Geometry check sheet. Reference: drawing and pictorial views, mm from the part's lowest x, y, z. A direction names the side the tool comes from. Round coordinates to 2 decimals unless told otherwise and drop trailing zeros. Loops run counter-clockwise (first coordinate to the right, second up) from the corner with the lowest first, then second, coordinate; pieces in that order, holes last. Notation, with made-up numbers: (45, -1.5) -> (92, -1.5) arc R14 ccw to (92, 16.5) -> close; hole circle Ø9 at (-35, 7). An arc over 180 degrees is marked (long way). Write item = value, one per line.
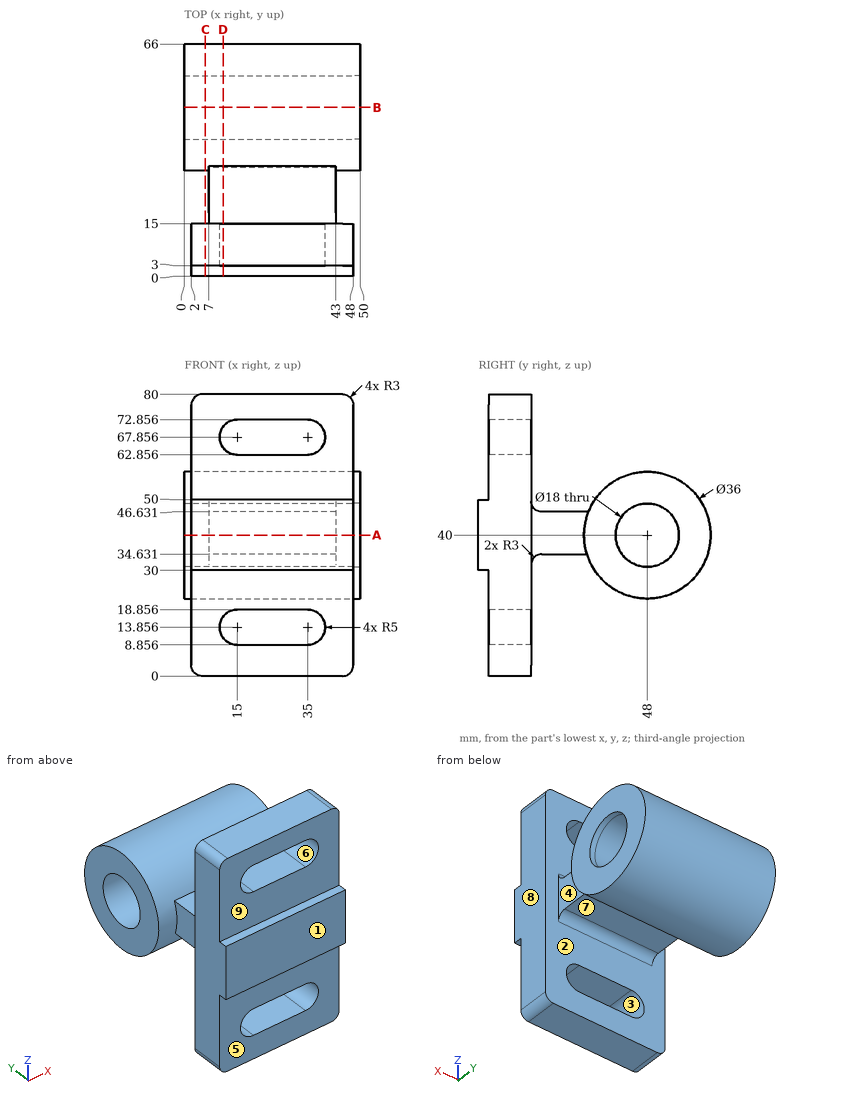
(1) Draft check along Y on the marked faces 1, 2, 3 and 4. Enter one of: released by +Y, released by -Y, zero draft, split by the parting line, or undercut.
Filled sheet:
face_1 = released by -Y
face_2 = undercut
face_3 = zero draft
face_4 = undercut
(2) Sectioned sample at A-A, the plane z = 40. Record the cut outline in (x, y), and give its area (3 significant figures).
Filled sheet:
outline = (0, 30) -> (7, 30) -> (7, 15) -> (2, 15) -> (2, 0) -> (48, 0) -> (48, 15) -> (43, 15) -> (43, 30) -> (50, 30) -> (50, 39) -> (0, 39) -> close; (0, 57) -> (50, 57) -> (50, 66) -> (0, 66) -> close
area = 2,130 mm2
(3) Set-up check for the marked faces 5, 6, 7, 8 and 9: record each of +Z, -Z, +X, -X, +Y, -Y from which the full face is reachable in a straight line by a thin tool's end or side.
Filled sheet:
face_5 = -Z, +X, -X, -Y
face_6 = +Y, -Y
face_7 = -Z, +X, -X
face_8 = +Z, -Z, +X, -Y
face_9 = +Z, +X, -X, -Y
(4) Sectioned sample at B-B, the plane y = 48. Record the cut outline in (x, z).
Filled sheet:
outline = (0, 22) -> (50, 22) -> (50, 31) -> (0, 31) -> close; (0, 49) -> (50, 49) -> (50, 58) -> (0, 58) -> close
(5) Material ranges on probe 1 along Y at (x, z) = (17, 40); probe 2 along Z at (x, y) = (17, 48); probe 3 along Y at (x, z) = (49.1, 40), recorded low to high. Write a range as from..to.
Filled sheet:
probe_1 = 0..39, 57..66
probe_2 = 22..31, 49..58
probe_3 = 30..39, 57..66
(6) Go/stop test with flat-tipped pins: pin 1 Ø13 at (y, z) = (22, 38.5) entering from -X; pin 2 Ø24 at (x, z) = (33.5, 21) entering from -Y; pin 3 Ø12 at (y, z) = (8.5, 41.5) entering from -X; pin 4 Ø23 at (x, z) = (34, 54) entering from +Y (1 decimal). Record where each tip stops, or that it passes through.
Filled sheet:
pin_1 = 7
pin_2 = 0
pin_3 = 2
pin_4 = 65.8
(7) Sectioned sample at C-C, the plane x = 6. Record the cut outline in (y, z), and give its area (3 significant figures).
Filled sheet:
outline = (0, 30) -> (3, 30) -> (3, 0) -> (15, 0) -> (15, 80) -> (3, 80) -> (3, 50) -> (0, 50) -> close; circle Ø36 at (48, 40); hole circle Ø18 at (48, 40)
area = 1,780 mm2
(8) Sectioned sample at D-D, the plane x = 11. Record the cut outline in (y, z) (1 decimal), and give its area (3 significant figures).
Filled sheet:
outline = (0, 30) -> (3, 30) -> (3, 16.9) -> (15, 16.9) -> (15, 31.6) arc R3 cw to (18, 34.6) -> (30.8, 34.6) arc R18 ccw (long way) to (31.3, 46.6) -> (18, 46.6) arc R3 cw to (15, 49.6) -> (15, 64.9) -> (3, 64.9) -> (3, 50) -> (0, 50) -> close; (3, 0) -> (15, 0) -> (15, 10.9) -> (3, 10.9) -> close; (3, 70.9) -> (15, 70.9) -> (15, 80) -> (3, 80) -> close; hole circle Ø18 at (48, 40)
area = 1,830 mm2
